from build123d import *

# Parameters (mm, degrees)
SKETCH_2_R      = 1.5
EXTRUDE_1_DEPTH = 1.5
FILLET_1_R      = 2


with BuildPart() as part:
    # ｽｹｯﾁ2 → ﾎﾞｽ - 押し出し1 (new body)
    with BuildSketch(Plane(origin=(0, 0, 0), x_dir=(1, 0, 0), z_dir=(0, 1, 0))):
        Polygon((0, 0), (30, 0), (30, 10), (10, 30), (0, 30), align=None)
        with Locations(Location((5, 5, 0), (0, 0, 270))):
            Circle(SKETCH_2_R, mode=Mode.SUBTRACT)
        with Locations(Location((25, 5, 0), (0, 0, 270))):
            Circle(SKETCH_2_R, mode=Mode.SUBTRACT)
        with Locations(Location((5, 25, 0), (0, 0, 90))):
            Circle(SKETCH_2_R, mode=Mode.SUBTRACT)
        with Locations(Location((5, 15, 0), (0, 0, 270))):
            Circle(SKETCH_2_R, mode=Mode.SUBTRACT)
        with Locations(Location((15, 5, 0), (0, 0, 270))):
            Circle(SKETCH_2_R, mode=Mode.SUBTRACT)
        with Locations(Location((15, 15, 0), (0, 0, 270))):
            Circle(SKETCH_2_R, mode=Mode.SUBTRACT)
    extrude(amount=EXTRUDE_1_DEPTH)

    # ﾌｨﾚｯﾄ1
    fillet_1_edges = [part.edges().sort_by_distance(p)[0] for p in [
        (0, 0.75, -30),
        (10, 0.75, -30),
        (30, 0.75, -10),
        (30, 0.75, 0),
        (0, 0.75, 0),
    ]]
    fillet(fillet_1_edges, radius=FILLET_1_R)


solid = part.part
Verification items for the finished model (mm, model axes). Round coordinates to 2 decimals unless told otherwise and drop trailing zeros. Loops run counter-clockwise (first coordinate to the right, second up) from the corner with the lowest first, then second, coordinate; pieces in that order, holes last. Notation, with made-up numbers: (70.5, -26.75) - (122.5, -26.75) arc R15 ccw to (122.5, -20.75) - close; hole circle Ø3 at (-21, 46.5). An arc over 180 degrees is marked (long way). Answer in a Markdown table with one row per item. Add a question column.
Q1. Section check A-A on z = -5. Enter the section's corners in (x, y), plus the area to 3 significant figures.
Q2. Gauge pin test, flat end, axial feed: pin 1 (3.5 mm diameter, centred on x = 5, z = -25, fed in from -Y). Record the tip position at first contact, or that the pin passes through.
Q3. Section check D-D on y = 0.45. Enter the section's corners in (x, z), plus the area to 3 significant figures.
Q4. Section check C-C on x = 25. Enter the section's corners in (y, z).
Q5. Material ranges on line 1 (X direction, y = 0.8, z = -5); line 2 (X direction, y = 0.15, z = -16); line 3 (X direction, y = 0.15, z = -15.5), recorded low to high.
Q6. Release check for a two-part mould opening along X. For faces 1 (the face through (6, 1, -30)), 2 (the face through (20, 1, -20)), 3 (the face through (16.01, 0.74, -6.11)), 4 (the face through (15.07, 0.74, -16.5)) record: pulls with the +X half, pulls with the -X half, needs draft (parallel to the pull), parting line crosses it, or undercut.
Q7. Section check B-B on x = 5. Enter the section's corners in (y, z).
Found:
| question | item | result |
|---|---|---|
| 1 | outline | (0, 0) - (3.5, 0) - (3.5, 1.5) - (0, 1.5) - close; (6.5, 0) - (13.5, 0) - (13.5, 1.5) - (6.5, 1.5) - close; (16.5, 0) - (23.5, 0) - (23.5, 1.5) - (16.5, 1.5) - close; (26.5, 0) - (30, 0) - (30, 1.5) - (26.5, 1.5) - close |
| 1 | area | 31.5 mm² |
| 2 | pin 1 | stops at y = 0 |
| 3 | outline | (0, -28) arc R2 ccw to (2, -30) - (9.17, -30) arc R2 ccw to (10.59, -29.41) - (29.41, -10.59) arc R2 ccw to (30, -9.17) - (30, -2) arc R2 ccw to (28, 0) - (2, 0) arc R2 ccw to (0, -2) - close; hole circle Ø3 at (5, -25); hole circle Ø3 at (5, -15); hole circle Ø3 at (5, -5); hole circle Ø3 at (15, -15); hole circle Ø3 at (15, -5); hole circle Ø3 at (25, -5) |
| 3 | area | 655 mm² |
| 4 | outline | (0, -15) - (1.5, -15) - (1.5, -6.5) - (0, -6.5) - close; (0, -3.5) - (1.5, -3.5) - (1.5, 0) - (0, 0) - close |
| 5 | line 1 | x = 0 to 3.5, 6.5 to 13.5, 16.5 to 23.5, 26.5 to 30 |
| 5 | line 2 | x = 0 to 3.88, 6.12 to 13.88, 16.12 to 24 |
| 5 | line 3 | x = 0 to 3.59, 6.41 to 13.59, 16.41 to 24.5 |
| 6 | face 1 | needs draft |
| 6 | face 2 | pulls with the +X half |
| 6 | face 3 | undercut |
| 6 | face 4 | undercut |
| 7 | outline | (0, -30) - (1.5, -30) - (1.5, -26.5) - (0, -26.5) - close; (0, -23.5) - (1.5, -23.5) - (1.5, -16.5) - (0, -16.5) - close; (0, -13.5) - (1.5, -13.5) - (1.5, -6.5) - (0, -6.5) - close; (0, -3.5) - (1.5, -3.5) - (1.5, 0) - (0, 0) - close |
